Part print with two shaded views. Sizes in mm from the minimum x, y, z corner. A direction names the side the tool comes from. Coordinates: 2 decimals unless noted, no trailing zeros. Loops run counter-clockwise (first coordinate to the right, second up) from the corner with the lowest first, then second, coordinate; pieces in that order, holes last. Notation, with made-up numbers: (58.5, 17.5) -> (87.5, 17.5) arc R21 cw to (87.5, 54.5) -> close; hole circle Ø7 at (61.25, 59.5). An arc over 180 degrees is marked (long way). Use one line per item in the form item = value.
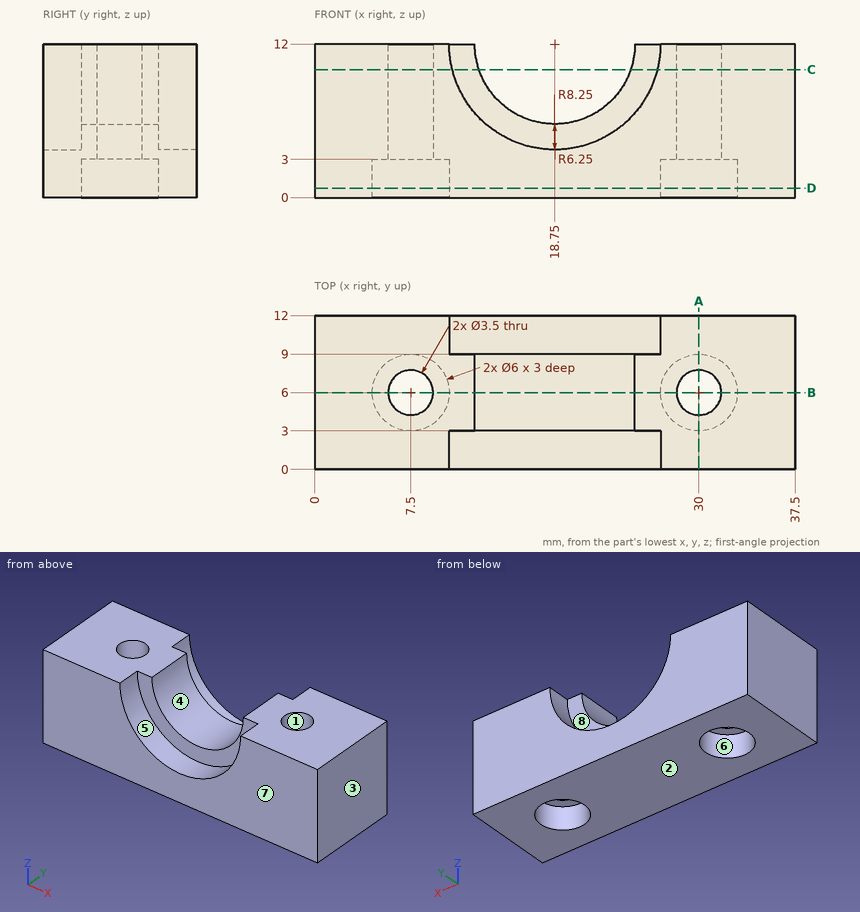
Q1. Pin check, flat tip, straight feed: pin 1 Ø4.5 at (x, y) = (7.5, 6) entering from -Z. Stop position of the tip, or through.
Result:
pin_1 = 3
Q2. Band-saw the part on A-A, the plane x = 30. Write the cut outline in (y, z).
Result:
outline = (0, 0) -> (3, 0) -> (3, 3) -> (4.25, 3) -> (4.25, 12) -> (0, 12) -> close; (7.75, 3) -> (9, 3) -> (9, 0) -> (12, 0) -> (12, 12) -> (7.75, 12) -> close
Q3. Wall check: line 1 along Y through (x, z) = (7.5, 8.25); line 2 along Y through (x, z) = (7.5, 2.75); line 3 along X through (y, z) = (6.75, 1.75). Give the ranges that are in metal, low to high.
Result:
line_1 = 0 to 4.25, 7.75 to 12
line_2 = 0 to 3, 9 to 12
line_3 = 0 to 4.6, 10.4 to 27.1, 32.9 to 37.5
Q4. Which spindle directions (+Z, -Z, +X, -X, +Y, -Y) get a long thin tool onto all of the face, cutting with end or side? Do the marked faces 5, 6, 7 and 8. Say none if no direction does.
Result:
face_5 = +Z, -Y
face_6 = -Z
face_7 = +Z, -Z, +X, -X, -Y
face_8 = +Z, +Y
Q5. Band-saw the part on C-C, the plane z = 10. Write the cut outline in (x, y), and give its area (3 significant figures).
Result:
outline = (0, 0) -> (10.75, 0) -> (10.75, 3) -> (12.83, 3) -> (12.83, 9) -> (10.75, 9) -> (10.75, 12) -> (0, 12) -> close; (24.67, 3) -> (26.75, 3) -> (26.75, 0) -> (37.5, 0) -> (37.5, 12) -> (26.75, 12) -> (26.75, 9) -> (24.67, 9) -> close; hole circle Ø3.5 at (7.5, 6); hole circle Ø3.5 at (30, 6)
area = 264 mm2
Q6. Mould opens along X. For the marked faces 1, 2, 3 and 4 say: released by +X, released by -X, zero draft, split by the parting line, or undercut.
Result:
face_1 = undercut
face_2 = zero draft
face_3 = released by +X
face_4 = undercut
Q7. Band-saw the part on B-B, the plane y = 6. Write the cut outline in (x, z).
Result:
outline = (0, 0) -> (4.5, 0) -> (4.5, 3) -> (5.75, 3) -> (5.75, 12) -> (0, 12) -> close; (9.25, 3) -> (10.5, 3) -> (10.5, 0) -> (27, 0) -> (27, 3) -> (28.25, 3) -> (28.25, 12) -> (25, 12) arc R6.25 cw to (12.5, 12) -> (9.25, 12) -> close; (31.75, 3) -> (33, 3) -> (33, 0) -> (37.5, 0) -> (37.5, 12) -> (31.75, 12) -> close
Q8. Band-saw the part on D-D, the plane z = 0.75. Write the cut outline in (x, y).
Result:
outline = (0, 0) -> (37.5, 0) -> (37.5, 12) -> (0, 12) -> close; hole circle Ø6 at (7.5, 6); hole circle Ø6 at (30, 6)
